from build123d import *

# Parameters (mm, degrees)
SKETCH2_R           = 8.25
SKETCH2_R_2         = 2
BOSS_EXTRUDE1_DEPTH = 2
BOSS_EXTRUDE2_DEPTH = 15


with BuildPart() as part:
    # Sketch2 → Boss-Extrude1 (new body)
    with BuildSketch(Plane(origin=(0, 0, 0), x_dir=(1, 0, 0), z_dir=(0, 1, 0))):
        with Locations(Location((0, 0, 0), (0, 0, 270))):
            Circle(SKETCH2_R)
        with Locations(Location((0, 0, 0), (0, 0, 270))):
            Circle(SKETCH2_R_2, mode=Mode.SUBTRACT)
    extrude(amount=BOSS_EXTRUDE1_DEPTH)

    # Sketch3 → Boss-Extrude2 (add)
    with BuildSketch(Plane(origin=(0, 2, 0), x_dir=(1, 0, 0), z_dir=(0, 1, 0))):
        with BuildLine():
            ThreePointArc((-4.836821281, 6.683386858), (-8.25, 0), (-4.836821281, -6.683386858))
            Line((-4.836821281, -6.683386858), (-4.836821281, -4.942960119))
            ThreePointArc((-4.836821281, -4.942960119), (-6.915756997, 0), (-4.836821281, 4.942960119))
            Line((-4.836821281, 4.942960119), (-4.836821281, 6.683386858))
        make_face()
        with BuildLine():
            Line((4.836821281, -4.942960119), (4.836821281, -6.683386858))
            ThreePointArc((4.836821281, -6.683386858), (7.34732181, -3.752247622), (8.25, 0))
            ThreePointArc((8.25, 0), (7.34732181, 3.752247622), (4.836821281, 6.683386858))
            Line((4.836821281, 6.683386858), (4.836821281, 4.942960119))
            ThreePointArc((4.836821281, 4.942960119), (6.374871585, 2.681176442), (6.915756997, 0))
            ThreePointArc((6.915756997, 0), (6.374871585, -2.681176442), (4.836821281, -4.942960119))
        make_face()
    extrude(amount=BOSS_EXTRUDE2_DEPTH)


solid = part.part
Verification items for the finished model (mm, model axes). A direction names the side the tool comes from. Coordinates: 2 decimals unless noted, no trailing zeros. Loops run counter-clockwise (first coordinate to the right, second up) from the corner with the lowest first, then second, coordinate; pieces in that order, holes last. Notation, with made-up numbers: (88, 72.25) -> (119, 72.25) arc R22 cw to (119, 90.25) -> close; hole circle Ø9 at (22.5, 21.5). An arc over 180 degrees is marked (long way). Answer as a JSON object with one key per item and string values. Group by question number.
Item 1: Sectioned sample at B-B on x = 0. Record the boundary of the cut face in (y, z).
Item 2: Tool access check on faces 3 (the flat face through (-4.837, 9, 6)), 4 (the flat face through (-2, 0, 2)). Record the directions out of +Z, -Z, +X, -X, +Y, -Y that give a thin tool (end or side, any length) a straight path to the whole face; none if there is none.
Item 3: Sectioned sample at C-C on z = 1.5. Record the boundary of the cut face in (x, y), plus the area to 3 significant figures.
Item 4: Mould release check, pull along X, two halves, no side actions. Record for faces 1 (the flat face through (7.3, 17, -0.1)), 2 (the cylindrical face through (-6.915, 9.395, 0.077)): +X half, -X half, draft (parallel to the pull), parting line (faces both ways), or undercut.
Item 5: Depth check by flat-ended pin: pin 1 (4.5 mm diameter, centred on x = 0, z = 0, fed in from +Y); pin 2 (1.9 mm diameter, centred on y = 11, z = -6, fed in from +X); pin 3 (8 mm diameter, centred on x = -5.5, y = 3, fed in from +Z); pin 4 (5 mm diameter, centred on x = -1, y = 5.5, fed in from +Z). Enter the tip coordinate at first touch or a pass-through.
Item 6: Sectioned sample at D-D on z = -4.25. Record the boundary of the cut face in (x, y).
Item 7: Sectioned sample at A-A on y = 16. Record the boundary of the cut face in (x, z).
Item 8: Scan lines: probe 1 along X at (y, z) = (0.5, 0); probe 2 along Y at (x, z) = (-5.75, -2.5); probe 3 along X at (y, z) = (15.25, -2.75). Record each from-to range of solid material in increasing order.
Evaluation:
{
 "1": {"outline": "(0, -8.25) -> (2, -8.25) -> (2, -2) -> (0, -2) -> close; (0, 2) -> (2, 2) -> (2, 8.25) -> (0, 8.25) -> close"},
 "2": {"face 3": "+Z, -Z, +Y", "face 4": "+Z, -Z, +X, -X, -Y"},
 "3": {"outline": "(-8.11, 0) -> (-1.32, 0) -> (-1.32, 2) -> (-6.75, 2) -> (-6.75, 17) -> (-8.11, 17) -> close; (1.32, 0) -> (8.11, 0) -> (8.11, 17) -> (6.75, 17) -> (6.75, 2) -> (1.32, 2) -> close", "area": "68.0 mm²"},
 "4": {"face 1": "draft", "face 2": "undercut"},
 "5": {"pin 1": "stops at y = 2", "pin 2": "stops at x = 6.52", "pin 3": "stops at z = 8.09", "pin 4": "passes through"},
 "6": {"outline": "(-7.07, 0) -> (7.07, 0) -> (7.07, 17) -> (5.46, 17) -> (5.46, 2) -> (-5.46, 2) -> (-5.46, 17) -> (-7.07, 17) -> close"},
 "7": {"outline": "(-4.84, -6.68) -> (-4.84, -4.94) arc R6.92 cw to (-4.84, 4.94) -> (-4.84, 6.68) arc R8.25 ccw to start; (4.84, -6.68) arc R8.25 ccw to (4.84, 6.68) -> (4.84, 4.94) arc R6.92 cw to (4.84, -4.94) -> close"},
 "8": {"probe 1": "x = -8.25 to -2, 2 to 8.25", "probe 2": "y = 0 to 2", "probe 3": "x = -7.78 to -6.35, 6.35 to 7.78"}
}
